The model under review builds one solid part; all positions refer to its coordinate system, in mm. A direction names the side the tool comes from. Round coordinates to 2 decimals unless told otherwise and drop trailing zeros. Order: outer loops, then holes, each group sorted by start corner. A loop starts at its lowest first (then second) coordinate and runs counter-clockwise, first axis right, second up. Notation, with made-up numbers: (86.5, 30) -> (138.5, 30) arc R13 ccw to (138.5, 46) -> close; hole circle Ø11 at (36.5, 14). An arc over 180 degrees is marked (long way). Put each result on its own line as item: value. Start each with the question number.
from build123d import *

# Parameters (mm, degrees)
SKETCH1_W           = 100
SKETCH1_H           = 180
BOSS_EXTRUDE1_DEPTH = 5
SKETCH2_R           = 2.1
CUT_EXTRUDE1_DEPTH  = 104.07764064
FILLET1_R           = 1.5
SKETCH3_R           = 2.1
CUT_EXTRUDE2_DEPTH  = 104.07764064


with BuildPart() as part:
    # Sketch1 → Boss-Extrude1 (new body)
    with BuildSketch(Plane.XY):
        Rectangle(SKETCH1_W, SKETCH1_H)
    extrude(amount=BOSS_EXTRUDE1_DEPTH)

    # Sketch2 → Cut-Extrude1 (cut, through all)
    with BuildSketch(Plane(origin=(0, 0, 0), x_dir=(-1, 0, 0), z_dir=(0, 0, -1))):
        with Locations((-22, -40)):
            Circle(SKETCH2_R)
        with Locations((0, -25)):
            Circle(SKETCH2_R)
        with Locations(Location((22, -40, 0), (0, 0, 180))):
            Circle(SKETCH2_R)
        with Locations(Location((0, -55, 0), (0, 0, 180))):
            Circle(SKETCH2_R)
        with BuildLine():
            Line((-10, -35), (10, -35))
            ThreePointArc((10, -35), (15, -40), (10, -45))
            Line((10, -45), (-10, -45))
            ThreePointArc((-10, -45), (-15, -40), (-10, -35))
        make_face()
    extrude(amount=-CUT_EXTRUDE1_DEPTH, mode=Mode.SUBTRACT)

    # Fillet1
    fillet1_edges = [part.edges().sort_by_distance(p)[0] for p in [
        (50, -90, 2.5),
        (-50, -90, 2.5),
        (-50, 90, 2.5),
        (50, 90, 2.5),
    ]]
    fillet(fillet1_edges, radius=FILLET1_R)

    # Sketch3 → Cut-Extrude2 (cut, through all)
    with BuildSketch(Plane(origin=(0, 0, 0), x_dir=(-1, 0, 0), z_dir=(0, 0, -1))):
        with Locations((-40, 75)):
            Circle(SKETCH3_R)
        with Locations((-40, 55)):
            Circle(SKETCH3_R)
        with Locations((-40, 35)):
            Circle(SKETCH3_R)
        with Locations((-40, 15)):
            Circle(SKETCH3_R)
        with Locations((-40, -5)):
            Circle(SKETCH3_R)
        with Locations(Location((40, -5, 0), (0, 0, 180))):
            Circle(SKETCH3_R)
        with Locations(Location((40, 15, 0), (0, 0, 180))):
            Circle(SKETCH3_R)
        with Locations(Location((40, 35, 0), (0, 0, 180))):
            Circle(SKETCH3_R)
        with Locations(Location((40, 75, 0), (0, 0, 180))):
            Circle(SKETCH3_R)
        with Locations(Location((40, 55, 0), (0, 0, 180))):
            Circle(SKETCH3_R)
        with Locations((-40, -25)):
            Circle(SKETCH3_R)
        with Locations((-40, -45)):
            Circle(SKETCH3_R)
        with Locations((-40, -65)):
            Circle(SKETCH3_R)
        with Locations(Location((40, -65, 0), (0, 0, 180))):
            Circle(SKETCH3_R)
        with Locations(Location((40, -45, 0), (0, 0, 180))):
            Circle(SKETCH3_R)
        with Locations(Location((40, -25, 0), (0, 0, 180))):
            Circle(SKETCH3_R)
    extrude(amount=-CUT_EXTRUDE2_DEPTH, mode=Mode.SUBTRACT)


solid = part.part
Q1. Wall thickness on probe 1 along Y at (x, z) = (9.5, 3.95); probe 2 along X at (y, z) = (-41.5, 3.35); probe 3 along X at (y, z) = (56, 1.5): over which ranges is each line inside the solid? List them lowest first. Write a range as [from, to].
Q2. Take a section at B-B on z = 1.1. State how many separate pieces and enclosed holes the cut face has, and give its area (3 significant figures).
Q3. Draft analysis for pull direction X (two halves, no side actions). For faces 3 (the face through (-1, 1, 5)), 4 (the face through (-50, -1, 2)), 5 (the face through (-42.1, -5.09, 2.46)), state which applies: +X half, -X half, draft (parallel to the pull), parting line (faces both ways), or undercut.
Q4. Take a section at D-D on x = -7. Give the boundary of the cut face in (y, z).
Q5. Take a section at C-C on y = -55. Give the boundary of the cut face in (x, z), and give its area (3 significant figures).
Q6. Take a section at A-A on y = 75. Give the boundary of the cut face in (x, z), and give its area (3 significant figures).
Q7. For faces 1 (the face through (-1, 90, 2)), 2 (the face through (0, -35, 2)), list the 3-axis set-ups (+Z, -Z, +X, -X, +Y, -Y) from which the entire face can be reached by the end or side of a thin tool; tool diameter is ignored.
Calculated:
1. probe 1: y = [-90, -45], [-35, 90]
1. probe 2: x = [-50, -23.47], [-20.53, -14.77], [14.77, 20.53], [23.47, 50]
1. probe 3: x = [-50, -41.85], [-38.15, 38.15], [41.85, 50]
2. separate pieces: 1
2. enclosed holes: 21
2. area: 17,400 mm²
3. face 3: draft
3. face 4: -X half
3. face 5: undercut
4. outline: (-90, 0) -> (-45, 0) -> (-45, 5) -> (-90, 5) -> close; (-35, 0) -> (90, 0) -> (90, 5) -> (-35, 5) -> close
5. outline: (-50, 0) -> (-2.1, 0) -> (-2.1, 5) -> (-50, 5) -> close; (2.1, 0) -> (50, 0) -> (50, 5) -> (2.1, 5) -> close
5. area: 479 mm²
6. outline: (-50, 0) -> (-42.1, 0) -> (-42.1, 5) -> (-50, 5) -> close; (-37.9, 0) -> (37.9, 0) -> (37.9, 5) -> (-37.9, 5) -> close; (42.1, 0) -> (50, 0) -> (50, 5) -> (42.1, 5) -> close
6. area: 458 mm²
7. face 1: +Z, -Z, +X, -X, +Y
7. face 2: +Z, -Z
